Part model, mm, in its own coordinate system. A direction names the side the tool comes from. Give positions to 0.01 mm unless a question says otherwise; leave off trailing zeros. Order: outer loops, then holes, each group sorted by start corner. A loop starts at its lowest first (then second) coordinate and runs counter-clockwise, first axis right, second up. Notation, with made-up numbers: (84.25, -6.5) - (135.25, -6.5) arc R14 ccw to (135.25, 20.5) - close; hole circle Ø8 at (27, 78.5). An arc over 180 degrees is marked (long way). One line per item, written item: value.
```python
from build123d import *

# Parameters (mm, degrees)
SKETCH1_W           = 99
SKETCH1_H           = 74
BOSS_EXTRUDE1_DEPTH = 30
SKETCH2_W           = 94
SKETCH2_H           = 69
CUT_EXTRUDE1_DEPTH  = 20
FILLET2_R           = 5
FILLET3_R           = 2
SKETCH3_R           = 2.5
BOSS_EXTRUDE2_DEPTH = 4
SKETCH8_R           = 1.45
CUT_EXTRUDE4_DEPTH  = 5
CHAMFER1_SIZE       = 2.5
CHAMFER1_SIZE2      = 3.19985408
CHAMFER2_SIZE       = 2.5
CHAMFER2_SIZE2      = 3.19985408
CHAMFER3_SIZE       = 2.5
CHAMFER3_SIZE2      = 3.19985408
CHAMFER4_SIZE       = 2.5
CHAMFER4_SIZE2      = 3.19985408
BOSS_EXTRUDE3_DEPTH = 30
SKETCH11_R          = 1.45
CUT_EXTRUDE5_DEPTH  = 6
FILLET5_R           = 2.5
SKETCH13_W          = 10
SKETCH13_H          = 4.8
CUT_EXTRUDE7_DEPTH  = 2.5
SKETCH14_W          = 7.6999997
SKETCH14_H          = 3.94999985
CUT_EXTRUDE8_DEPTH  = 2.5


with BuildPart() as part:
    # Sketch1 → Boss-Extrude1 (new body)
    with BuildSketch(Plane(origin=(0, 0, 0), x_dir=(1, 0, 0), z_dir=(0, 1, 0))):
        Rectangle(SKETCH1_W, SKETCH1_H)
    extrude(amount=BOSS_EXTRUDE1_DEPTH)

    # Sketch2 → Cut-Extrude1 (cut)
    with BuildSketch(Plane(origin=(0, 30, 0), x_dir=(1, 0, 0), z_dir=(0, 1, 0))):
        Rectangle(SKETCH2_W, SKETCH2_H)
    extrude(amount=-CUT_EXTRUDE1_DEPTH, mode=Mode.SUBTRACT)

    # Fillet2
    fillet2_edges = [part.edges().sort_by_distance(p)[0] for p in [
        (49.5, 15, 37),
        (-49.5, 15, 37),
        (-49.5, 15, -37),
        (49.5, 15, -37),
    ]]
    fillet(fillet2_edges, radius=FILLET2_R)

    # Fillet3
    fillet3_edges = [part.edges().sort_by_distance(p)[0] for p in [
        (47, 20, -34.5),
        (47, 20, 34.5),
        (-47, 20, 34.5),
        (-47, 20, -34.5),
    ]]
    fillet(fillet3_edges, radius=FILLET3_R)

    # Sketch3 → Boss-Extrude2 (add)
    with BuildSketch(Plane(origin=(0, 10, 0), x_dir=(1, 0, 0), z_dir=(0, 1, 0))):
        with Locations(Location((-36.255, 29.1465, 0), (0, 0, 270))):
            Circle(SKETCH3_R)
        with Locations(Location((41.469, 29.1465, 0), (0, 0, 270))):
            Circle(SKETCH3_R)
        with Locations(Location((41.471, -28.8925, 0), (0, 0, 270))):
            Circle(SKETCH3_R)
        with Locations(Location((-36.763, -28.8925, 0), (0, 0, 270))):
            Circle(SKETCH3_R)
    extrude(amount=BOSS_EXTRUDE2_DEPTH)

    # Sketch8 → Cut-Extrude4 (cut)
    with BuildSketch(Plane(origin=(0, 14, 0), x_dir=(1, 0, 0), z_dir=(0, 1, 0))):
        with Locations(Location((-36.255, 29.1465, 0), (0, 0, 270))):
            Circle(SKETCH8_R)
        with Locations(Location((-36.763, -28.8925, 0), (0, 0, 270))):
            Circle(SKETCH8_R)
        with Locations(Location((41.469, 29.1465, 0), (0, 0, 270))):
            Circle(SKETCH8_R)
        with Locations(Location((41.471, -28.8925, 0), (0, 0, 270))):
            Circle(SKETCH8_R)
    extrude(amount=-CUT_EXTRUDE4_DEPTH, mode=Mode.SUBTRACT)

    # Chamfer1
    chamfer1_edges = [part.edges().sort_by_distance(p)[0] for p in [
        (-36.763, 10, 26.3925),
    ]]
    chamfer1_side = [part.faces().sort_by_distance(p)[0] for p in [
        (-0.030421175, 10, 0.001557545),
    ]]
    chamfer(chamfer1_edges, length=CHAMFER1_SIZE, length2=CHAMFER1_SIZE2, reference=chamfer1_side[0])

    # Chamfer2
    chamfer2_edges = [part.edges().sort_by_distance(p)[0] for p in [
        (41.471, 10, 26.3925),
    ]]
    chamfer2_side = [part.faces().sort_by_distance(p)[0] for p in [
        (0.310585286, 10, -0.266651178),
    ]]
    chamfer(chamfer2_edges, length=CHAMFER2_SIZE, length2=CHAMFER2_SIZE2, reference=chamfer2_side[0])

    # Chamfer3
    chamfer3_edges = [part.edges().sort_by_distance(p)[0] for p in [
        (-36.255, 10, -31.6465),
    ]]
    chamfer3_side = [part.faces().sort_by_distance(p)[0] for p in [
        (-0.075107512, 10, -0.53988639),
    ]]
    chamfer(chamfer3_edges, length=CHAMFER3_SIZE, length2=CHAMFER3_SIZE2, reference=chamfer3_side[0])

    # Chamfer4
    chamfer4_edges = [part.edges().sort_by_distance(p)[0] for p in [
        (41.469, 10, -31.6465),
    ]]
    chamfer4_side = [part.faces().sort_by_distance(p)[0] for p in [
        (0.267122265, 10, -0.269293132),
    ]]
    chamfer(chamfer4_edges, length=CHAMFER4_SIZE, length2=CHAMFER4_SIZE2, reference=chamfer4_side[0])

    # Sketch10 → Boss-Extrude3 (add)
    with BuildSketch(Plane.XZ):
        with BuildLine():
            Line((-2.5, 37), (2.5, 37))
            ThreePointArc((2.5, 37), (0, 39.5), (-2.5, 37))
        make_face()
        with BuildLine():
            Line((-49.5, -2.5), (-49.5, 2.5))
            ThreePointArc((-49.5, 2.5), (-52, 0), (-49.5, -2.5))
        make_face()
        with BuildLine():
            Line((-2.5, -37), (2.5, -37))
            ThreePointArc((2.5, -37), (0, -39.5), (-2.5, -37))
        make_face()
        with BuildLine():
            Line((49.5, 2.5), (49.5, -2.5))
            ThreePointArc((49.5, -2.5), (52, 0), (49.5, 2.5))
        make_face()
    extrude(amount=-BOSS_EXTRUDE3_DEPTH)

    # Sketch11 → Cut-Extrude5 (cut)
    with BuildSketch(Plane(origin=(0, 30, 0), x_dir=(1, 0, 0), z_dir=(0, 1, 0))):
        with Locations(Location((0, 37, 0), (0, 0, 270))):
            Circle(SKETCH11_R)
        with Locations(Location((-49.5, 0, 0), (0, 0, 270))):
            Circle(SKETCH11_R)
        with Locations(Location((0, -37, 0), (0, 0, 270))):
            Circle(SKETCH11_R)
        with Locations(Location((49.5, 0, 0), (0, 0, 270))):
            Circle(SKETCH11_R)
    extrude(amount=-CUT_EXTRUDE5_DEPTH, mode=Mode.SUBTRACT)

    # Fillet5
    fillet5_edges = [part.edges().sort_by_distance(p)[0] for p in [
        (2.5, 15, 37),
        (-2.5, 15, 37),
        (-2.5, 15, -37),
        (2.5, 15, -37),
        (-49.5, 15, 2.5),
        (-49.5, 15, -2.5),
        (49.5, 15, -2.5),
        (49.5, 15, 2.5),
    ]]
    fillet(fillet5_edges, radius=FILLET5_R)

    # Sketch13 → Cut-Extrude7 (cut)
    with BuildSketch(Plane.ZY.offset(49.5)):
        with Locations((21.37405504, 18)):
            Rectangle(SKETCH13_W, SKETCH13_H)
    extrude(amount=-CUT_EXTRUDE7_DEPTH, mode=Mode.SUBTRACT)

    # Sketch14 → Cut-Extrude8 (cut)
    with BuildSketch(Plane.XY.offset(37)):
        with Locations((28.33814532, 21.075027895)):
            Rectangle(SKETCH14_W, SKETCH14_H)
    extrude(amount=-CUT_EXTRUDE8_DEPTH, mode=Mode.SUBTRACT)


solid = part.part
```
1) Cut at A-A, the plane z = -6. Give the cut face in (x, y), then the cut area to 3 significant figures.
Outcome:
outline: (-49.5, 0) - (49.5, 0) - (49.5, 30) - (47, 30) - (47, 10) - (-47, 10) - (-47, 30) - (-49.5, 30) - close
area: 1,090 mm^2
2) Pin check, flat tips, straight feed: pin 1 (8 mm diameter, centred on y = 24, z = 11.5, fed in from +X); pin 2 (5.5 mm diameter, centred on x = -36, z = 28.5, fed in from +Y); pin 3 (6 mm diameter, centred on x = -40, y = 24.5, fed in from -Z). Stop position of each tip, or through.
Outcome:
pin 1: stops at x = 49.5
pin 2: stops at y = 14
pin 3: stops at z = -37
3) Drill centre lines: line 1 along Z through (x, y) = (35.5, 25); line 2 along X through (y, z) = (20.5, 24.5); line 3 along Y through (x, z) = (26, -32.5). Where is each one in solid material? Low to high. Write a range as from..to.
Outcome:
line 1: z = -37..-34.5, 34.5..37
line 2: x = -49.5..-47, 47..49.5
line 3: y = 0..10
4) Which spindle directions (+Z, -Z, +X, -X, +Y, -Y) get a long thin tool onto all of the face, cutting with end or side? Do faces 1 (the flat face through (0, 30, 35)), 2 (the cylindrical face through (-35.073, 13.594, 27.05)), 3 (the flat face through (49.5, 15, -18)), 4 (the flat face through (32.188, 21, 36)). Say none if no direction does.
Outcome:
face 1: +Z, -Z, +X, -X, +Y
face 2: +Y
face 3: -Z, +X, +Y, -Y
face 4: +Z
5) Cut at B-B, the plane x = 0. Give the cut face in (y, z), then the cut area to 3 significant figures.
Outcome:
outline: (0, -39.5) - (30, -39.5) - (30, -38.45) - (24, -38.45) - (24, -35.55) - (30, -35.55) - (30, -34.5) - (10, -34.5) - (10, 34.5) - (30, 34.5) - (30, 35.55) - (24, 35.55) - (24, 38.45) - (30, 38.45) - (30, 39.5) - (0, 39.5) - close
area: 955 mm^2
6) Cut at C-C, the plane y = 7.25. Give the cut face in (x, z).
Outcome:
outline: (-50.75, -2.17) arc R2.5 cw to (-49.5, -4.33) - (-49.5, -32) arc R5 ccw to (-44.5, -37) - (-4.33, -37) arc R2.5 cw to (-2.17, -38.25) arc R2.5 ccw to (2.17, -38.25) arc R2.5 cw to (4.33, -37) - (44.5, -37) arc R5 ccw to (49.5, -32) - (49.5, -4.33) arc R2.5 cw to (50.75, -2.17) arc R2.5 ccw to (50.75, 2.17) arc R2.5 cw to (49.5, 4.33) - (49.5, 32) arc R5 ccw to (44.5, 37) - (4.33, 37) arc R2.5 cw to (2.17, 38.25) arc R2.5 ccw to (-2.17, 38.25) arc R2.5 cw to (-4.33, 37) - (-44.5, 37) arc R5 ccw to (-49.5, 32) - (-49.5, 4.33) arc R2.5 cw to (-50.75, 2.17) arc R2.5 ccw to start
7) Mould opens along X. For faces 5 (the cylindrical face through (48, 15.21, 35.57)), 6 (the conical face through (40.467, 13.044, 31.314)), 7 (the flat face through (-1, 0, -1)) say: released by +X, released by -X, zero draft, split by the parting line, or undercut.
Outcome:
face 5: released by +X
face 6: undercut
face 7: zero draft
